Source: three-view drawing plus pictorial views. Frame: mm from the lowest corner of the part. Round coordinates to 2 decimals unless told otherwise and drop trailing zeros. Write each loop counter-clockwise with the first axis right and the second up, starting at its lowest first coordinate (ties: lowest second). Pieces come first, ordered by that corner, then holes.
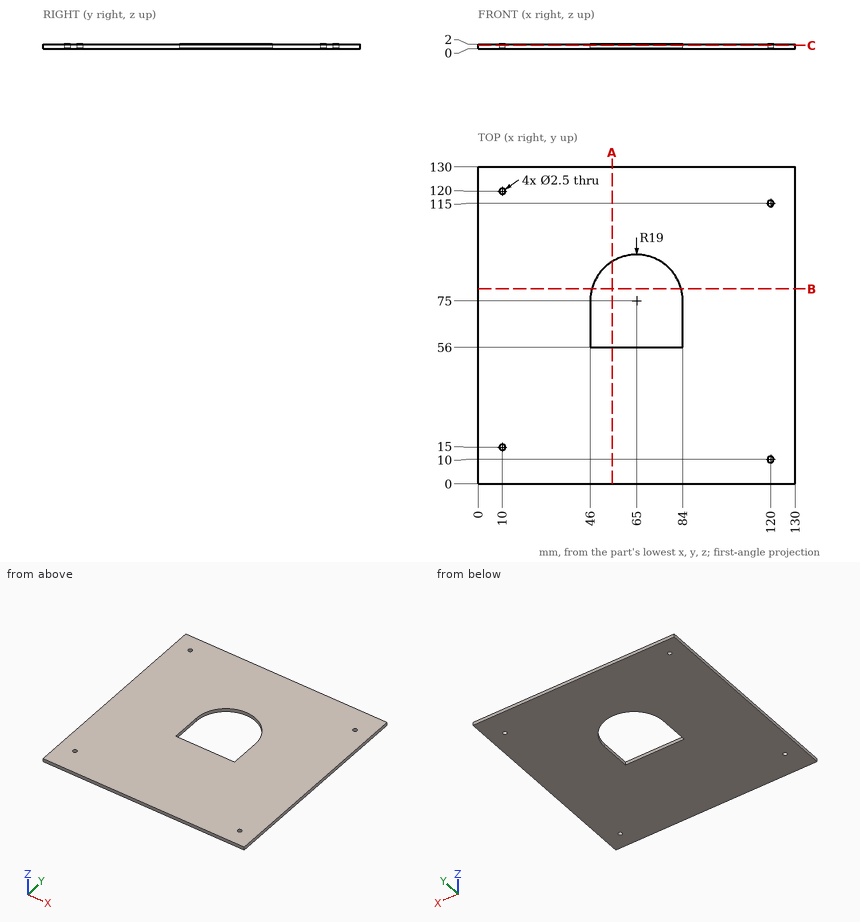
1) Section A-A on x = 55. Output: boundary loops of the cut face in (y, z), plus the area to 3 significant figures.
2) Section B-B on y = 80. Output: boundary loops of the cut face in (x, z).
3) Line query: probe 1 along Y at (x, z) = (10, 1.5); probe 2 along Y at (x, z) = (120, 0.8); probe 3 along X at (y, z) = (120, 0.8). Output: solid intervals per line, ascending.
4) First-contact query: P1, Ø4, axis at x = 120, y = 115, coming from the +Z side. Flat tip, straight axial feed; report the tip coordinate or a pass-through.
5) Section C-C on z = 1.45. Output: boundary loops of the cut face in (x, y), plus the area to 3 significant figures.
Filled in:
1. outline: (0, 0) - (56, 0) - (56, 2) - (0, 2) - close; (91.16, 0) - (130, 0) - (130, 2) - (91.16, 2) - close
1. area: 190 mm2
2. outline: (0, 0) - (46.67, 0) - (46.67, 2) - (0, 2) - close; (83.33, 0) - (130, 0) - (130, 2) - (83.33, 2) - close
3. probe 1: y = 0 to 13.75, 16.25 to 118.75, 121.25 to 130
3. probe 2: y = 0 to 8.75, 11.25 to 113.75, 116.25 to 130
3. probe 3: x = 0 to 8.75, 11.25 to 130
4. P1: stops at z = 2
5. outline: (0, 0) - (130, 0) - (130, 130) - (0, 130) - close; hole circle Ø2.5 at (10, 15); hole circle Ø2.5 at (10, 120); hole (46, 56) - (84, 56) - (84, 75) arc R19 ccw to (46, 75) - close; hole circle Ø2.5 at (120, 10); hole circle Ø2.5 at (120, 115)
5. area: 15,600 mm2
